For this review, take the finished solid that the model builds, in its own axes (mm). Face numbers are marked on the shaded views. A direction names the side the tool comes from. Give positions to 0.01 mm unless a question says otherwise; leave off trailing zeros. Order: outer loops, then holes, each group sorted by start corner. A loop starts at its lowest first (then second) coordinate and runs counter-clockwise, first axis right, second up. Notation, with made-up numbers: (-3.5, 22) -> (35.5, 22) arc R14 ccw to (35.5, 45) -> close; hole circle Ø7 at (31.5, -15). An arc over 180 degrees is marked (long way). One line per item, written item: value. Start each with the question number.
from build123d import *

# Parameters (mm, degrees)
M3X0_5_TAPPED_HOLE1_REACH           = 32.48
M3X0_5_TAPPED_HOLE1_BORE_R          = 1.25
M3X0_5_TAPPED_HOLE1_ON_FACE_2_REACH = 32.48
M3X0_5_TAPPED_HOLE1_BORE_2_R        = 1.25
CHAMFER1_SIZE                       = 0.508


with BuildPart() as part:
    # Sketch1 → Revolve1 (revolve)
    with BuildSketch(Plane.XY, mode=Mode.PRIVATE) as revolve1_sk:
        Polygon((-0.381, 1.0033), (-3.0988, 5.710667685), (-3.0988, 9.525), (-7.1628, 9.525), (-7.1628, 15.24), (0, 15.24), (0, 13.1445), (3.048, 13.1445), (3.048, 10.795), (0, 10.795), (0, 1.0033), align=None)
    revolve(revolve1_sk.sketch.rotate(Axis((0, 0, 0), (-1, 0, 0)), 90), axis=Axis((0, 0, 0), (-1, 0, 0)))  # turned: the seam where the file's is

    # M3x0.5 Tapped Hole1 bore (on position points) → M3x0.5 Tapped Hole1 (cut, up to next)
    with BuildSketch(Plane(origin=(-5.1308, 15.24, 0), x_dir=(0, 0, 1), z_dir=(0, 1, 0)), mode=Mode.PRIVATE) as m3x0_5_tapped_hole1_sk1:
        Circle(M3X0_5_TAPPED_HOLE1_BORE_R)
    m3x0_5_tapped_hole1_tool1 = extrude(m3x0_5_tapped_hole1_sk1.sketch, amount=-M3X0_5_TAPPED_HOLE1_REACH, mode=Mode.PRIVATE) & part.part
    add(m3x0_5_tapped_hole1_tool1.solids().sort_by_distance((-5.1308, 15.24, 0))[0], mode=Mode.SUBTRACT)

    # M3x0.5 Tapped Hole1 bore 2 (on position points) → M3x0.5 Tapped Hole1 on face 2 (cut, up to next)
    with BuildSketch(Plane(origin=(-5.1308, 0, 15.24), x_dir=(1, 0, 0), z_dir=(0, 0, 1)), mode=Mode.PRIVATE) as m3x0_5_tapped_hole1_on_face_2_sk1:
        Circle(M3X0_5_TAPPED_HOLE1_BORE_2_R)
    m3x0_5_tapped_hole1_on_face_2_tool1 = extrude(m3x0_5_tapped_hole1_on_face_2_sk1.sketch, amount=-M3X0_5_TAPPED_HOLE1_ON_FACE_2_REACH, mode=Mode.PRIVATE) & part.part
    add(m3x0_5_tapped_hole1_on_face_2_tool1.solids().sort_by_distance((-5.1308, 0, 15.24))[0], mode=Mode.SUBTRACT)

    # Chamfer1
    chamfer1_edges = [part.edges().sort_by_distance(p)[0] for p in [
        (-7.1628, 0, 15.24),
        (0, 0, 15.24),
        (3.048, 0, 13.1445),
    ]]
    chamfer(chamfer1_edges, length=CHAMFER1_SIZE)


solid = part.part
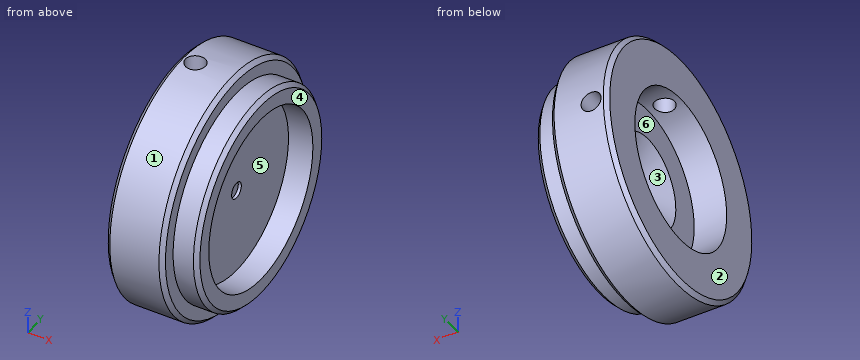
Q1. For the marked faces 4, 5 and 6, list the 3-axis set-ups (+Z, -Z, +X, -X, +Y, -Y) from which the entire face can be reached by the end or side of a thin tool; tool diameter is ignored.
Q2. Take a section at C-C (x = 1.75). State the section outline as (y, z) points (1 decimal), and give its area (3 significant figures).
Q3. For line 1 along Y through (x, z) = (1.6, 0) (1 decimal); line 2 along X through (y, z) = (0, 13.5); line 3 along Z through (x, y) = (-1.75, -2), list the stretches that pass through material, from the lowest coordinate up.
Q4. For pin 1 Ø9 at (y, z) = (-0.5, -1) entering from +X; pin 2 Ø3 at (x, z) = (-6, 2.5) entering from +Y; pin 3 Ø2 at (y, z) = (-2.5, -3) entering from -X; pin 4 Ø1.2 at (y, z) = (0, 0) entering from -X, all flat-tipped, find the tip position at first contact; note any pin that passes through.
Q5. Take a section at D-D (x = -5.5). State the section outline as (y, z) points (3 decimals).
Q6. Take a section at A-A (z = 0). State how many separate pieces and enclosed holes the cut face has, and give its area (3 significant figures).
Q7. Mouldability with a two-part tool opening along Z and no side actions: class the marked faces 1, 2 and 3 as pulls with the +Z half, pulls with the -Z half, needs draft (parallel to the pull), parting line crosses it, or undercut.
Answers below:
1. face 4: +Z, -Z, +X, +Y, -Y
1. face 5: +X
1. face 6: -X
2. outline: circle Ø26.3 at (0, 0); hole circle Ø21.6 at (0, 0)
2. area: 177 mm²
3. line 1: y = -13.1 to -10.8, 10.8 to 13.1
3. line 2: x = -7.16 to -6.38, -3.88 to 0
3. line 3: z = -15.11 to -2.72, 2.72 to 15.11
4. pin 1: stops at x = 0
4. pin 2: stops at y = 15.21
4. pin 3: stops at x = -2.63
4. pin 4: passes through
5. outline: (-1.194, 9.45) -> (-1.194, 15.193) arc R15.24 ccw (long way) to (15.193, -1.194) -> (9.45, -1.194) arc R9.525 cw (long way) to start; (1.194, 9.45) arc R9.525 cw to (9.45, 1.194) -> (15.193, 1.194) arc R15.24 ccw to (1.194, 15.193) -> close
6. separate pieces: 3
6. enclosed holes: 0
6. area: 121 mm²
7. face 1: parting line crosses it
7. face 2: needs draft
7. face 3: undercut
